```python
from build123d import *


with BuildPart() as part:
    # Esquisse1 → Révolution1 (revolve)
    with BuildSketch(Plane(origin=(0, 0, 0), x_dir=(0, 0, -1), z_dir=(1, 0, 0))):
        with BuildLine():
            Line((10.5, 23.354104043), (10.5, 21.613435))
            ThreePointArc((10.5, 21.613435), (7.595227269, 19.104514548), (6, 15.613435))
            Line((6, 15.613435), (6, 5.613435))
            Line((6, 5.613435), (3, 5.613435))
            Line((3, 5.613435), (3, -9.386565))
            Line((3, -9.386565), (2.386565, -10))
            Line((2.386565, -10), (0, -10))
            Line((0, -10), (0, 26.613435))
            ThreePointArc((0, 26.613435), (5.319852473, 25.892936282), (10.256410256, 23.783351967))
            ThreePointArc((10.256410256, 23.783351967), (10.434859246, 23.600878101), (10.5, 23.354104043))
        make_face()
    revolve(axis=Axis((0, -10, 0), (0, 1, 0)))


solid = part.part
```
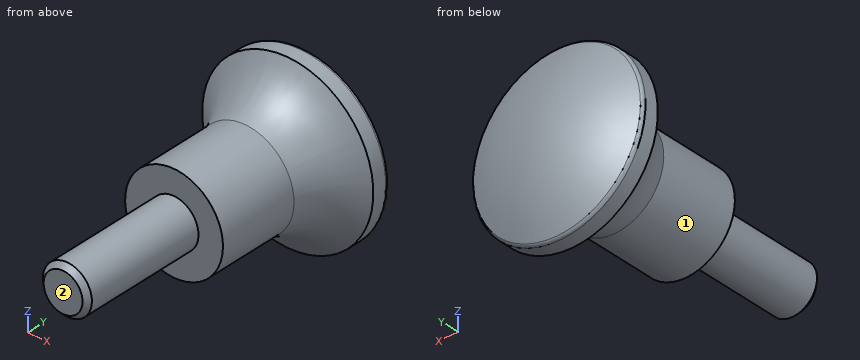
Work out the finished part from the listing and answer in its coordinate system (mm). Face numbers are marked on the shaded views. A direction names the side the tool comes from. Give positions to 0.01 mm unless a question says otherwise; leave off trailing zeros. Loops run counter-clockwise (first coordinate to the right, second up) from the corner with the lowest first, then second, coordinate; pieces in that order, holes last. Notation, with made-up numbers: (5, 31) - (59, 31) arc R13 cw to (59, 44) - close; hole circle Ø8 at (76.5, -9.75). An arc over 180 degrees is marked (long way). One line per question, with ' | ' between items.
(1) A tool of negligible diameter and unlimited length cuts with its end or side. For the marked faces 1 and 2, from which of +Z, -Z, +X, -X, +Y, -Y can it reach the whole face along a straight path? Write none if from no direction.
Recorded:
face 1: -Y | face 2: +Z, -Z, +X, -X, -Y
(2) Each of these flat-tipped pins is pushed along its axis until it touches: pin 1 Ø5 at (y, z) = (3.5, 1) entering from +X; pin 2 Ø3 at (x, y) = (-5.5, 6) entering from -Z; pin 3 Ø5 at (x, z) = (-3.5, 6) entering from +Y. Where does it stop, or does it pass through?
Recorded:
pin 1: stops at x = 6 | pin 2: stops at z = -4.47 | pin 3: stops at y = 26.11
(3) The part is cut by section B-B (x = 0). Write down the section's boundary in (y, z).
Recorded:
outline: (-10, -2.39) - (-9.39, -3) - (5.61, -3) - (5.61, -6) - (15.61, -6) arc R9 cw to (21.61, -10.5) - (23.35, -10.5) arc R0.5 ccw to (23.78, -10.26) arc R20 ccw to (23.78, 10.26) arc R0.5 ccw to (23.35, 10.5) - (21.61, 10.5) arc R9 cw to (15.61, 6) - (5.61, 6) - (5.61, 3) - (-9.39, 3) - (-10, 2.39) - close
(4) The part is cut by section A-A (z = 0). Write down the section's boundary in (x, y).
Recorded:
outline: (-10.5, 21.61) arc R9 cw to (-6, 15.61) - (-6, 5.61) - (-3, 5.61) - (-3, -9.39) - (-2.39, -10) - (2.39, -10) - (3, -9.39) - (3, 5.61) - (6, 5.61) - (6, 15.61) arc R9 cw to (10.5, 21.61) - (10.5, 23.35) arc R0.5 ccw to (10.26, 23.78) arc R20 ccw to (-10.26, 23.78) arc R0.5 ccw to (-10.5, 23.35) - close
(5) The part is cut by section D-D (y = 8). Write down the section's boundary in (x, z).
Recorded:
outline: circle Ø12 at (0, 0)
(6) The part is cut by section C-C (y = 1). Write down the section's boundary in (x, z).
Recorded:
outline: circle Ø6 at (0, 0)
(7) Straight lines are drawn through the part: probe 1 along Y at (x, z) = (-3, 1.75); probe 2 along X at (y, z) = (4, 1.75); probe 3 along Z at (x, y) = (-2, -4). For each, find the intervals that lie inside material, in ascending order.
Recorded:
probe 1: y = 5.61 to 26.31 | probe 2: x = -2.44 to 2.44 | probe 3: z = -2.24 to 2.24
